CAD build for the part. Positions are in the model's coordinates, mm. Round coordinates to 2 decimals unless told otherwise and drop trailing zeros. Loops run counter-clockwise (first coordinate to the right, second up) from the corner with the lowest first, then second, coordinate; pieces in that order, holes last. Notation, with made-up numbers: (-16.5, 37.25) - (2.5, 37.25) arc R21 cw to (2.5, 61.25) - close; hole circle Ø1 at (-15.75, -18). An arc over 180 degrees is marked (long way). Use one line per item in the form item = value.
from build123d import *

# Parameters (mm, degrees)
F1_DEPTH      = 12.7
F1_DEPTH_BACK = 12.7


with BuildPart() as f1:
    # F0 (on Top) → F1 (new body, two sides)
    with BuildSketch(Plane.XY) as f1_sk:
        with BuildLine():
            ThreePointArc((-111.9032161657, 45.1075771975), (-104.9388147825, 49.6046967237), (-102.233028536, 57.4408750939))
            ThreePointArc((-102.233028536, 57.4408750939), (-103.1495920186, 62.1780286527), (-105.7669850463, 66.2314181228))
            ThreePointArc((-105.7669850463, 66.2314181228), (-111.3902737379, 69.6367304735), (-117.9628407751, 69.7741730225))
            ThreePointArc((-117.9628407751, 69.7741730225), (-123.7235718813, 66.6069182803), (-127.1288839844, 60.9836296554))
            ThreePointArc((-127.1288839844, 60.9836296554), (-124.0990716757, 48.6503316999), (-111.9032161657, 45.1075771975))
        make_face()
        with BuildLine():
            ThreePointArc((-119.0629153027, 66.3050093604), (-118.9416645433, 67.8436709883), (-117.720455796, 68.7875091882))
            ThreePointArc((-117.720455796, 68.7875091882), (-116.2009205472, 68.5169653295), (-115.3805191431, 67.2096310616))
            ThreePointArc((-115.3805191431, 67.2096310616), (-113.4541917392, 67.1074092571), (-111.5854100251, 66.6290354813))
            ThreePointArc((-111.5854100251, 66.6290354813), (-109.4453537915, 67.6632905836), (-107.9625390148, 65.8056618162))
            ThreePointArc((-107.9625390148, 65.8056618162), (-108.0598650939, 65.2045461904), (-108.3418985903, 64.6648523252))
            ThreePointArc((-108.3418985903, 64.6648523252), (-107.0520611513, 63.2304514239), (-106.0688942695, 61.5707618605))
            ThreePointArc((-106.0688942695, 61.5707618605), (-104.3354570915, 61.3284924248), (-103.531389131, 59.773830518))
            ThreePointArc((-103.531389131, 59.773830518), (-103.9963531849, 58.526705234), (-105.1642725683, 57.8883657009))
            ThreePointArc((-105.1642725683, 57.8883657009), (-105.1565898795, 57.6646790168), (-105.154028536, 57.4408750939))
            ThreePointArc((-105.154028536, 57.4408750939), (-105.3028711794, 55.7411956283), (-105.7448681486, 54.0932565829))
            ThreePointArc((-105.7448681486, 54.0932565829), (-104.956169881, 53.3903974367), (-104.6632418137, 52.3753855727))
            ThreePointArc((-104.6632418137, 52.3753855727), (-105.7150762613, 50.6721141497), (-107.7090513047, 50.8497451481))
            ThreePointArc((-107.7090513047, 50.8497451481), (-109.143452206, 49.5599077092), (-110.8031417694, 48.5767408274))
            ThreePointArc((-110.8031417694, 48.5767408274), (-110.7222846244, 48.2650711548), (-110.6950731119, 47.9442356888))
            ThreePointArc((-110.6950731119, 47.9442356888), (-112.4636646746, 46.0441257609), (-114.485537929, 47.6721191262))
            ThreePointArc((-114.485537929, 47.6721191262), (-116.4118653329, 47.7743409307), (-118.280647047, 48.2527147064))
            ThreePointArc((-118.280647047, 48.2527147064), (-120.9853017302, 47.4465844645), (-121.5241584818, 50.2168978626))
            ThreePointArc((-121.5241584818, 50.2168978626), (-122.8139959207, 51.6512987638), (-123.7971628025, 53.3109883272))
            ThreePointArc((-123.7971628025, 53.3109883272), (-126.2796626303, 54.6534478339), (-124.7017845037, 56.9933844868))
            ThreePointArc((-124.7017845037, 56.9933844868), (-124.5995626992, 58.9197118907), (-124.1211889235, 60.7884936048))
            ThreePointArc((-124.1211889235, 60.7884936048), (-124.9273191654, 63.493148288), (-122.1570057673, 64.0320050396))
            ThreePointArc((-122.1570057673, 64.0320050396), (-120.7226048661, 65.3218424786), (-119.0629153027, 66.3050093604))
        make_face(mode=Mode.SUBTRACT)
        with BuildLine():
            ThreePointArc((-105.7669850463, 66.2314181228), (-103.1495920186, 62.1780286527), (-102.233028536, 57.4408750939))
            ThreePointArc((-102.233028536, 57.4408750939), (-104.9388147825, 49.6046967237), (-111.9032161657, 45.1075771975))
            ThreePointArc((-111.9032161657, 45.1075771975), (-97.0154400661, 46.358254472), (-82.4698502509, 42.9471127619))
            ThreePointArc((-82.4698502509, 42.9471127619), (-80.4804099193, 42.9769764127), (-79.1228638065, 44.4315668094))
            ThreePointArc((-79.1228638065, 44.4315668094), (-78.3454622215, 46.8126113043), (-77.7261887634, 49.2395901865))
            ThreePointArc((-77.7261887634, 49.2395901865), (-78.0931330297, 51.1951250433), (-79.7569486957, 52.2862172026))
            ThreePointArc((-79.7569486957, 52.2862172026), (-93.8663258144, 57.199011108), (-105.7669850463, 66.2314181228))
        make_face()
        with BuildLine():
            ThreePointArc((-136.9851331378, 29.5548252922), (-125.675840017, 39.3175075021), (-111.9032161657, 45.1075771975))
            ThreePointArc((-111.9032161657, 45.1075771975), (-124.0990716757, 48.6503316999), (-127.1288839844, 60.9836296554))
            ThreePointArc((-127.1288839844, 60.9836296554), (-133.4896537424, 47.4650986561), (-143.7165840545, 36.5738191773))
            ThreePointArc((-143.7165840545, 36.5738191773), (-144.6854415401, 34.8359814855), (-144.1045023609, 32.9330168666))
            ThreePointArc((-144.1045023609, 32.9330168666), (-142.4311581332, 31.0692450977), (-140.6389694958, 29.3194491099))
            ThreePointArc((-140.6389694958, 29.3194491099), (-138.7619544987, 28.6594647379), (-136.9851331378, 29.5548252922))
        make_face()
        with BuildLine():
            ThreePointArc((-111.5854100251, 66.6290354813), (-113.4541917392, 67.1074092571), (-115.3805191431, 67.2096310616))
            ThreePointArc((-115.3805191431, 67.2096310616), (-115.3658740322, 67.0739229362), (-115.3609839601, 66.9375144989))
            ThreePointArc((-115.3609839601, 66.9375144989), (-115.7668519034, 65.7620877354), (-116.8115121243, 65.0875198096))
            ThreePointArc((-116.8115121243, 65.0875198096), (-118.1721404496, 65.2618339158), (-119.0629153027, 66.3050093604))
            ThreePointArc((-119.0629153027, 66.3050093604), (-120.7226048661, 65.3218424786), (-122.1570057673, 64.0320050396))
            ThreePointArc((-122.1570057673, 64.0320050396), (-121.5945438354, 63.3595301674), (-121.3928152584, 62.5063646151))
            ThreePointArc((-121.3928152584, 62.5063646151), (-122.2828033944, 60.8942926824), (-124.1211889235, 60.7884936048))
            ThreePointArc((-124.1211889235, 60.7884936048), (-124.5995626992, 58.9197118907), (-124.7017845037, 56.9933844868))
            ThreePointArc((-124.7017845037, 56.9933844868), (-123.182542657, 56.5479556158), (-122.5246679411, 55.1079196698))
            ThreePointArc((-122.5246679411, 55.1079196698), (-122.8750060343, 54.0069876303), (-123.7971628025, 53.3109883272))
            ThreePointArc((-123.7971628025, 53.3109883272), (-122.8139959207, 51.6512987638), (-121.5241584818, 50.2168978626))
            ThreePointArc((-121.5241584818, 50.2168978626), (-119.3974024314, 50.8837622924), (-118.0935180572, 49.0760883715))
            ThreePointArc((-118.0935180572, 49.0760883715), (-118.1408892899, 48.6539031482), (-118.280647047, 48.2527147064))
            ThreePointArc((-118.280647047, 48.2527147064), (-116.4118653329, 47.7743409307), (-114.485537929, 47.6721191262))
            ThreePointArc((-114.485537929, 47.6721191262), (-113.0545449478, 49.7942303781), (-110.8031417694, 48.5767408274))
            ThreePointArc((-110.8031417694, 48.5767408274), (-109.143452206, 49.5599077092), (-107.7090513047, 50.8497451481))
            ThreePointArc((-107.7090513047, 50.8497451481), (-108.1977457206, 53.3621692456), (-105.7448681486, 54.0932565829))
            ThreePointArc((-105.7448681486, 54.0932565829), (-105.3028711794, 55.7411956283), (-105.154028536, 57.4408750939))
            ThreePointArc((-105.154028536, 57.4408750939), (-105.1565898795, 57.6646790168), (-105.1642725683, 57.8883657009))
            ThreePointArc((-105.1642725683, 57.8883657009), (-107.2863838203, 59.3193586821), (-106.0688942695, 61.5707618605))
            ThreePointArc((-106.0688942695, 61.5707618605), (-107.0520611513, 63.2304514239), (-108.3418985903, 64.6648523252))
            ThreePointArc((-108.3418985903, 64.6648523252), (-110.8543226878, 64.1761579093), (-111.5854100251, 66.6290354813))
        make_face()
        with BuildLine():
            ThreePointArc((-117.9628407751, 69.7741730225), (-111.3902737379, 69.6367304735), (-105.7669850463, 66.2314181228))
            ThreePointArc((-105.7669850463, 66.2314181228), (-114.2939916511, 78.4992719445), (-118.6126513027, 92.8016933424))
            ThreePointArc((-118.6126513027, 92.8016933424), (-119.6332341487, 94.5096673835), (-121.5717194408, 94.9580416056))
            ThreePointArc((-121.5717194408, 94.9580416056), (-122.8013442638, 94.7195500651), (-124.0224652534, 94.4407688797))
            Line((-124.0224652534, 94.4407688797), (-117.9628407751, 69.7741730225))
        make_face()
        with BuildLine():
            ThreePointArc((-127.1288839844, 60.9836296554), (-123.7235718813, 66.6069182803), (-117.9628407751, 69.7741730225))
            Line((-117.9628407751, 69.7741730225), (-124.0224652534, 94.4407688797))
            ThreePointArc((-124.0224652534, 94.4407688797), (-125.2337626594, 94.1219993476), (-126.4339273489, 93.7635859852))
            ThreePointArc((-126.4339273489, 93.7635859852), (-127.9439980797, 92.4680355004), (-128.0570037746, 90.4815827868))
            ThreePointArc((-128.0570037746, 90.4815827868), (-125.2569195337, 75.8061065896), (-127.1288839844, 60.9836296554))
        make_face()
    extrude(amount=F1_DEPTH)
    extrude(f1_sk.sketch, amount=-F1_DEPTH_BACK)


solid = f1.part
1) Slice it at B-B (y = 39). Write the cut outline in (x, z), plus the area to 3 significant figures.
Report:
outline = (-140.83, -12.7) - (-126.18, -12.7) - (-126.18, 12.7) - (-140.83, 12.7) - close
area = 372 mm^2
2) Flat gauge pins, fed straight in: pin 1 (5 mm diameter, centred on x = -96, z = 5.5, fed in from -Y); pin 2 (1.5 mm diameter, centred on x = -131, z = 9.5, fed in from -Y); pin 3 (3 mm diameter, centred on x = -120, y = 49.08, fed in from +Z); pin 4 (4 mm diameter, centred on y = 50, z = 5, fed in from -X). Where does each tip first touch, or does it go through?
Report:
pin_1 = 45.97
pin_2 = 34.85
pin_3 = through
pin_4 = -133.13
3) Slice it at A-A (z = 4.25). State how many separate pieces and enclosed holes the cut face has, plus the area to 3 significant figures.
Report:
separate_pieces = 1
enclosed_holes = 8
area = 1,290 mm^2
4) Slice it at C-C (x = -92). Write the cut outline in (y, z).
Report:
outline = (45.72, -12.7) - (56.25, -12.7) - (56.25, 12.7) - (45.72, 12.7) - close
5) Two-plate mould, pull along X, no slides. Class faces 1 (the cylindrical face through (-142.455, 31.095, 0.178)), 2 (the flat face through (-114, 57, 12.7)), 3 (the cylindrical face through (-80.507, 42.966, 0.178)): +X half, -X half, draft (parallel to the pull), parting line (faces both ways), or undercut.
Report:
face_1 = -X half
face_2 = draft
face_3 = undercut
6) Drill centre lines: probe 1 along Y at (x, z) = (-107.5, 5.25); probe 2 along X at (y, z) = (47, 5.5); probe 3 along Y at (x, z) = (-111, 9). Where is each one in solid material? Low to high.
Report:
probe_1 = 45.97 to 50.71, 54.04 to 68.14
probe_2 = -133.81 to -114.25, -110.95 to -78.29
probe_3 = 45.32 to 46.91, 48.98 to 64.27, 67.34 to 72.74
